Verification items for the finished model (mm, model axes). A direction names the side the tool comes from. Give positions to 0.01 mm unless a question says otherwise; leave off trailing zeros. Write each loop counter-clockwise with the first axis right and the second up, starting at its lowest first coordinate (ties: lowest second). Pieces come first, ordered by that corner, then holes. Notation, with made-up numbers: (-14.75, 62) - (5.25, 62) arc R19 cw to (5.25, 97) - close; hole circle Ø5 at (-16.5, -7.5). An arc over 180 degrees is marked (long way). Put each result on its own line as item: value.
from build123d import *

# Parameters (mm, degrees)
F0_R     = 6
F0_R_2   = 2.6
F1_DEPTH = 25
F2_DEPTH = 18


with BuildPart() as f1:
    # F0 (on Top) → F1 (new body)
    with BuildSketch(Plane.XY):
        with Locations((-2.922279, 4.134713)):
            Circle(F0_R)
        with Locations((-2.922279, 4.134713)):
            Circle(F0_R_2, mode=Mode.SUBTRACT)
    extrude(amount=F1_DEPTH)

    # F0 (on Top) → F2 (join)
    with BuildSketch(Plane.XY):
        with BuildLine():
            ThreePointArc((-34.729826, 56.185457), (-52.177662, 43.41457), (-60.745847, 23.562398))
            ThreePointArc((-60.745847, 23.562398), (-62.392882, 17.70849), (-63.448871, 11.719679))
            ThreePointArc((-63.448871, 11.719679), (-64.342738, -9.884106), (-54.16386, -28.960609))
            ThreePointArc((-54.16386, -28.960609), (-50.613999, -33.898165), (-46.590157, -38.457733))
            ThreePointArc((-46.590157, -38.457733), (-30.256955, -52.626326), (-8.995918, -56.562165))
            ThreePointArc((-8.995918, -56.562165), (-2.922279, -56.865287), (3.15136, -56.562165))
            ThreePointArc((3.15136, -56.562165), (24.412397, -52.626326), (40.745599, -38.457733))
            ThreePointArc((40.745599, -38.457733), (44.769441, -33.898165), (48.319302, -28.960609))
            ThreePointArc((48.319302, -28.960609), (58.498179, -9.884106), (57.604313, 11.719679))
            ThreePointArc((57.604313, 11.719679), (56.548324, 17.70849), (54.901289, 23.562398))
            ThreePointArc((54.901289, 23.562398), (46.333104, 43.41457), (28.885268, 56.185457))
            ThreePointArc((28.885268, 56.185457), (23.544629, 59.093814), (17.94095, 61.455963))
            ThreePointArc((17.94095, 61.455963), (-2.922279, 67.134713), (-23.785508, 61.455963))
            ThreePointArc((-23.785508, 61.455963), (-29.389187, 59.093814), (-34.729826, 56.185457))
        make_face()
        with BuildLine():
            Line((-26.641882, -37.019029), (-7.189733, -10.245442))
            ThreePointArc((-7.189733, -10.245442), (-2.922279, -10.865287), (1.345175, -10.245442))
            Line((1.345175, -10.245442), (20.797324, -37.019029))
            ThreePointArc((20.797324, -37.019029), (-2.922279, -43.365287), (-26.641882, -37.019029))
        make_face(mode=Mode.SUBTRACT)
        with BuildLine():
            Line((-49.391573, 13.976191), (-17.917334, 3.74959))
            ThreePointArc((-17.917334, 3.74959), (-17.188127, -0.500542), (-15.279903, -4.367589))
            Line((-15.279903, -4.367589), (-34.732052, -31.141176))
            ThreePointArc((-34.732052, -31.141176), (-48.097464, -10.543594), (-49.391573, 13.976191))
        make_face(mode=Mode.SUBTRACT)
        with Locations((-2.922279, 4.134713)):
            Circle(F0_R, mode=Mode.SUBTRACT)
        with BuildLine():
            Line((28.887494, -31.141176), (9.435345, -4.367589))
            ThreePointArc((9.435345, -4.367589), (11.343569, -0.500542), (12.072776, 3.74959))
            Line((12.072776, 3.74959), (43.547015, 13.976191))
            ThreePointArc((43.547015, 13.976191), (42.252905, -10.543594), (28.887494, -31.141176))
        make_face(mode=Mode.SUBTRACT)
        with BuildLine():
            ThreePointArc((-46.301403, 23.486756), (-30.842079, 42.56302), (-7.922279, 51.370822))
            Line((-7.922279, 51.370822), (-7.922279, 18.276848))
            ThreePointArc((-7.922279, 18.276848), (-11.739058, 16.269968), (-14.827164, 13.260156))
            Line((-14.827164, 13.260156), (-46.301403, 23.486756))
        make_face(mode=Mode.SUBTRACT)
        with BuildLine():
            ThreePointArc((8.982606, 13.260156), (5.8945, 16.269968), (2.077721, 18.276848))
            Line((2.077721, 18.276848), (2.077721, 51.370822))
            ThreePointArc((2.077721, 51.370822), (24.99752, 42.56302), (40.456845, 23.486756))
            Line((40.456845, 23.486756), (8.982606, 13.260156))
        make_face(mode=Mode.SUBTRACT)
    extrude(amount=F2_DEPTH)


solid = f1.part
Q1. Section check C-C, the plane y = 32. Record the cut outline in (x, z).
Answers follow:
outline: (-58.61, 0) - (-41.39, 0) - (-41.39, 18) - (-58.61, 18) - close; (-7.92, 0) - (2.08, 0) - (2.08, 18) - (-7.92, 18) - close; (35.55, 0) - (52.77, 0) - (52.77, 18) - (35.55, 18) - close
Q2. Section check D-D, the plane x = 46. Record the cut outline in (y, z).
Answers follow:
outline: (-32.3, 0) - (43.83, 0) - (43.83, 18) - (-32.3, 18) - close
Q3. Set-up check for faces 1 (the face through (-3.007, -56.865, 8.874)), 2 (the face through (11.325, -0.558, 8.874)): record each of +Z, -Z, +X, -X, +Y, -Y from which the full face is reachable in a straight line by a thin tool's end or side.
Answers follow:
face 1: +Z, -Z, -Y
face 2: +Z, -Z
Q4. Release check for a two-part mould opening along Y. For faces 3 (the face through (-11.7, 16.3, 8.9)), 4 (the face through (-51.99, 43.65, 8.87)), 5 (the face through (0, 3, 25)) record: released by +Y, released by -Y, zero draft, split by the parting line, or undercut.
Answers follow:
face 3: undercut
face 4: released by +Y
face 5: zero draft
Q5. Go/stop test with flat-tipped pins: pin 1 Ø2 at (y, z) = (47, 15) entering from -X; pin 2 Ø14.5 at (y, z) = (29.5, 6) entering from -X; pin 3 Ø10 at (y, z) = (5.5, 21) entering from -X. Record where each tip stops, or that it passes through.
Answers follow:
pin 1: stops at x = -49.93
pin 2: stops at x = -61.17
pin 3: stops at x = -65.31
Q6. Section check B-B, the plane z = 22. Record the cut outline in (x, y), plus the area to 3 significant figures.
Answers follow:
outline: circle Ø12 at (-2.92, 4.13); hole circle Ø5.2 at (-2.92, 4.13)
area: 91.9 mm2
Q7. Section check A-A, the plane y = -8. Record the cut outline in (x, z), plus the area to 3 significant figures.
Answers follow:
outline: (-64.73, 0) - (-48.85, 0) - (-48.85, 18) - (-64.73, 18) - close; (-17.92, 0) - (12.07, 0) - (12.07, 18) - (-17.92, 18) - close; (43, 0) - (58.88, 0) - (58.88, 18) - (43, 18) - close
area: 1,110 mm2
Q8. Scan lines: line 1 along X through (y, z) = (-21.5, 16.5); line 2 along X through (y, z) = (25, 10.5); line 3 along Y through (x, z) = (-19.5, 2.5). Record each from-to range of solid material in increasing order.
Answers follow:
line 1: x = -59.75 to -42.91, -27.73 to -15.37, 9.52 to 21.88, 37.07 to 53.9
line 2: x = -60.51 to -45.59, -7.92 to 2.08, 39.75 to 54.67
line 3: y = -56.09 to -40.38, -27.19 to -10.18, 4.26 to 14.78, 48.65 to 63.65
